For this review, take the finished solid that the model builds, in its own axes (mm). A direction names the side the tool comes from. Give positions to 0.01 mm unless a question says otherwise; leave off trailing zeros. Write each loop counter-clockwise with the first axis right and the second up, starting at its lowest first coordinate (ties: lowest second). Pieces come first, ordered by that corner, then holes. Notation, with made-up numbers: (-35.5, -24) -> (3.5, -24) arc R24 ccw to (3.5, -9) -> close; hole circle Ø3 at (46, -33.5). An arc over 180 degrees is marked (long way). Return JSON: item names as keys, results as strings.
from build123d import *

# Parameters (mm, degrees)
CUT_EXTRUDE_1_DEPTH = 0.5


with BuildPart() as part:
    # 草图1 → 旋转1 (revolve)
    with BuildSketch(Plane.XY, mode=Mode.PRIVATE) as revolve_1_sk:
        with BuildLine():
            Line((1.5, 2.5), (1.5, 1.5))
            Line((1.5, 1.5), (8.283239619, 1.5))
            Line((8.283239619, 1.5), (11.5, 0))
            Line((11.5, 0), (0, 0))
            ThreePointArc((0, 0), (0.126225608, 1.274754878), (0.5, 2.5))
            Line((0.5, 2.5), (1.5, 2.5))
        make_face()
    revolve(revolve_1_sk.sketch.rotate(Axis((-93.852509653, 0, 0), (1, 0, 0)), 90), axis=Axis((-93.852509653, 0, 0), (1, 0, 0)))

    # 草图2 → 切除-拉伸1 (cut)
    with BuildSketch(Plane(origin=(0, 0, 0), x_dir=(0, 0, -1), z_dir=(1, 0, 0))):
        with BuildLine():
            Line((1.5, 0.25), (1.05, 0.25))
            ThreePointArc((1.05, 0.25), (0.484314575, 0.484314575), (0.25, 1.05))
            Line((0.25, 1.05), (0.25, 1.5))
            Line((0.25, 1.5), (-0.25, 1.5))
            Line((-0.25, 1.5), (-0.25, 1.05))
            ThreePointArc((-0.25, 1.05), (-0.484314575, 0.484314575), (-1.05, 0.25))
            Line((-1.05, 0.25), (-1.5, 0.25))
            Line((-1.5, 0.25), (-1.5, -0.25))
            Line((-1.5, -0.25), (-1.05, -0.25))
            ThreePointArc((-1.05, -0.25), (-0.484314575, -0.484314575), (-0.25, -1.05))
            Line((-0.25, -1.05), (-0.25, -1.5))
            Line((-0.25, -1.5), (0.25, -1.5))
            Line((0.25, -1.5), (0.25, -1.05))
            ThreePointArc((0.25, -1.05), (0.484314575, -0.484314575), (1.05, -0.25))
            Line((1.05, -0.25), (1.5, -0.25))
            Line((1.5, -0.25), (1.5, 0.25))
        make_face()
    extrude(amount=CUT_EXTRUDE_1_DEPTH, mode=Mode.SUBTRACT)


solid = part.part
1. Add section A-A, the plane x = 5.25. State the section outline as (y, z) points, plus the area to 3 significant figures.
Results found:
{"outline": "circle Ø3 at (0, 0)", "area": "7.07 mm²"}
2. Add section D-D, the plane z = 1.65. State the section outline as (x, y) points.
Results found:
{"outline": "(0.5, -1.88) -> (1.5, -1.88) -> (1.5, 1.88) -> (0.5, 1.88) arc R6.29 ccw to start"}
3. To check wall thickness, follow probe 1 along Z at (x, y) = (0.75, -2); probe 2 along Z at (x, y) = (6, 0.9). State the ranges of each line that lie inside material, in increasing order.
Results found:
{"probe 1": "z = -1.5 to 1.5", "probe 2": "z = -1.2 to 1.2"}
4. Add section B-B, the plane z = -1.8. State the section outline as (x, y) points.
Results found:
{"outline": "(0.5, -1.73) -> (1.5, -1.73) -> (1.5, 1.73) -> (0.5, 1.73) arc R6.25 ccw to start"}
5. The part is to be moulded in two halves that separate along Y. For faces 1 (the cylindrical face through (0.26, -0.49, -0.48)), 2 (the flat face through (1.5, 0, 2)), 3 (the conical face through (10.27, -0.17, 0.55)), say which applies: +Y half, -Y half, draft (parallel to the pull), parting line (faces both ways), or undercut.
Results found:
{"face 1": "undercut", "face 2": "draft", "face 3": "parting line"}
6. For faces 4 (the cylindrical face through (4.94, -0.45, 1.43)), 5 (the cylindrical face through (1, -0.1, -2.5)), 6 (the cylindrical face through (0.26, -0.48, 0.49)), list the 3-axis set-ups (+Z, -Z, +X, -X, +Y, -Y) from which the entire face can be reached by the end or side of a thin tool; tool diameter is ignored.
Results found:
{"face 4": "+X", "face 5": "+X, -X", "face 6": "-X"}
7. For pin 1 (1 mm diameter, centred on y = -1.5, z = 0, fed in from +X); pin 2 (1.5 mm diameter, centred on x = 5.5, z = 1.5, fed in from -Y); pin 3 (0.5 mm diameter, centred on x = 0.5, z = -1, fed in from +Y), all flat-tipped, find the tip position at first contact; note any pin that passes through.
Results found:
{"pin 1": "stops at x = 9.36", "pin 2": "stops at y = -1.3", "pin 3": "stops at y = 2.38"}
8. Add section C-C, the plane x = 1.25. State the section outline as (y, z) points, plus the area to 3 significant figures.
Results found:
{"outline": "circle Ø5 at (0, 0)", "area": "19.6 mm²"}
